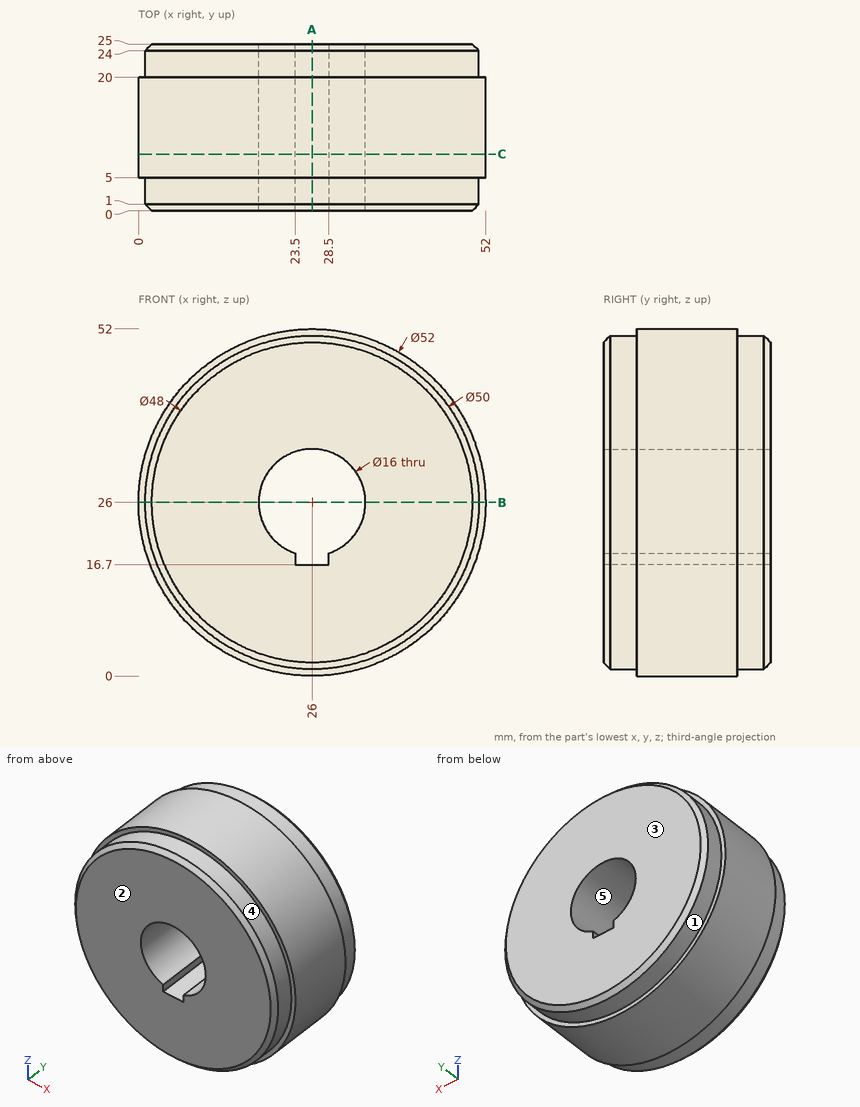
For this review, use the dimensioned drawing (mm, ordinates from the lowest corner) and the shaded views. A direction names the side the tool comes from. Round coordinates to 2 decimals unless told otherwise and drop trailing zeros. Order: outer loops, then holes, each group sorted by start corner. A loop starts at its lowest first (then second) coordinate and runs counter-clockwise, first axis right, second up. Notation, with made-up numbers: (59, 74) -> (103, 74) arc R23 ccw to (103, 108) -> close; hole circle Ø1 at (83.25, 20). An arc over 180 degrees is marked (long way). One line per item, written item: value. Start each with the question number.
Q1. Take a section at A-A (x = 26). Write out the cut boundary in (y, z).
Q2. Clearance check with flat-ended pins moving along their axes: pin 1 Ø4 at (x, y) = (12.5, 2.5) entering from -Z; pin 2 Ø3 at (x, y) = (29, 10) entering from +Z; pin 3 Ø12 at (y, z) = (15, 32) entering from -X. State where each tip first meets the part, or that it passes through.
Q3. Mouldability with a two-part tool opening along X and no side actions: class the marked faces 3, 4 and 5 as released by +X, released by -X, zero draft, split by the parting line, or undercut.
Q4. Take a section at B-B (z = 26). Write out the cut boundary in (x, y), and give its area (3 significant figures).
Q5. Machinability: for the marked faces 1 and 2, which of the approach directions +Z, -Z, +X, -X, +Y, -Y give a long, thin tool a straight path to every point of the face, cutting with its end or side? Answer none if there is none.
Q6. Take a section at C-C (y = 8.5). Write out the cut boundary in (x, z), and give its area (3 significant figures).
Q7. Wall thickness on line 1 (X direction, y = 9.5, z = 26); line 2 (Z direction, x = 29, y = 7); line 3 (X direction, y = 3.75, z = 29): over which ranges is each line inside the solid? List them lowest first.
Reported:
1. outline: (0, 2) -> (1, 1) -> (5, 1) -> (5, 0) -> (20, 0) -> (20, 1) -> (24, 1) -> (25, 2) -> (25, 16.7) -> (0, 16.7) -> close; (0, 34) -> (25, 34) -> (25, 50) -> (24, 51) -> (20, 51) -> (20, 52) -> (5, 52) -> (5, 51) -> (1, 51) -> (0, 50) -> close
2. pin 1: stops at z = 3.8
2. pin 2: stops at z = 51.96
2. pin 3: stops at x = 0
3. face 3: zero draft
3. face 4: split by the parting line
3. face 5: undercut
4. outline: (0, 5) -> (1, 5) -> (1, 1) -> (2, 0) -> (18, 0) -> (18, 25) -> (2, 25) -> (1, 24) -> (1, 20) -> (0, 20) -> close; (34, 0) -> (50, 0) -> (51, 1) -> (51, 5) -> (52, 5) -> (52, 20) -> (51, 20) -> (51, 24) -> (50, 25) -> (34, 25) -> close
4. area: 878 mm2
5. face 1: +Y
5. face 2: +Z, -Z, +X, -X, -Y
6. outline: circle Ø52 at (26, 26); hole (23.5, 16.7) -> (28.5, 16.7) -> (28.5, 18.4) arc R8 ccw (long way) to (23.5, 18.4) -> close
6. area: 1,920 mm2
7. line 1: x = 0 to 18, 34 to 52
7. line 2: z = 0.17 to 18.58, 33.42 to 51.83
7. line 3: x = 1.18 to 18.58, 33.42 to 50.82
